```python
from build123d import *

# Parameters (mm, degrees)
SKETCH_1_R          = 5
EXTRUDE_1_DEPTH     = 14
SKETCH_2_R          = 2.5
CUT_EXTRUDE_1_DEPTH = 7
SKETCH_3_W          = 1
SKETCH_3_H          = 14
CUT_EXTRUDE_2_DEPTH = 14
SKETCH_4_R          = 2
CUT_EXTRUDE_3_DEPTH = 10
SKETCH_5_R          = 3
CUT_EXTRUDE_4_DEPTH = 2


with BuildPart() as part:
    # 草图1 → 凸台-拉伸1 (new body)
    with BuildSketch(Plane.XY):
        Polygon((21, 0), (-21, 0), (-21, 6), (-9, 6), (-9, 32.8), (9, 32.8), (9, 6), (21, 6), align=None)
        with Locations((0, 20)):
            Circle(SKETCH_1_R, mode=Mode.SUBTRACT)
    extrude(amount=EXTRUDE_1_DEPTH)

    # 草图2 → 切除-拉伸1 (cut, through all)
    with BuildSketch(Plane(origin=(0, 6, 0), x_dir=(1, 0, 0), z_dir=(0, 1, 0))):
        with Locations((-16, -7)):
            Circle(SKETCH_2_R)
        with Locations((16, -7)):
            Circle(SKETCH_2_R)
    extrude(amount=-CUT_EXTRUDE_1_DEPTH, mode=Mode.SUBTRACT)

    # 草图3 → 切除-拉伸2 (cut)
    with BuildSketch(Plane(origin=(0, 32.8, 0), x_dir=(1, 0, 0), z_dir=(0, 1, 0))):
        with Locations((0, -7)):
            Rectangle(SKETCH_3_W, SKETCH_3_H)
    extrude(amount=-CUT_EXTRUDE_2_DEPTH, mode=Mode.SUBTRACT)

    # 草图4 → 切除-拉伸3 (cut, symmetric)
    with BuildSketch(Plane(origin=(-0.5, 0, 0), x_dir=(0, 0, -1), z_dir=(1, 0, 0))):
        with Locations((-7, 28.887468593)):
            Circle(SKETCH_4_R)
    extrude(amount=CUT_EXTRUDE_3_DEPTH, both=True, mode=Mode.SUBTRACT)

    # 草图5 → 切除-拉伸4 (cut)
    with BuildSketch(Plane(origin=(9, 0, 0), x_dir=(0, 0, -1), z_dir=(1, 0, 0))):
        with Locations((-7, 28.887468593)):
            Circle(SKETCH_5_R)
    extrude(amount=-CUT_EXTRUDE_4_DEPTH, mode=Mode.SUBTRACT)


solid = part.part
```
For this review, take the finished solid that the model builds, in its own axes (mm). A direction names the side the tool comes from. Round coordinates to 2 decimals unless told otherwise and drop trailing zeros. Write each loop counter-clockwise with the first axis right and the second up, starting at its lowest first coordinate (ties: lowest second). Pieces come first, ordered by that corner, then holes. Notation, with made-up numbers: (41.25, 17) -> (99.25, 17) arc R12 ccw to (99.25, 22) -> close; hole circle Ø3 at (-36.5, 40.25). An arc over 180 degrees is marked (long way). Use one line per item in the form item = value.
Q1. Consider section B-B (y = 20). State the section outline as (x, z) points.
Resolved:
outline = (-9, 0) -> (-5, 0) -> (-5, 14) -> (-9, 14) -> close; (5, 0) -> (9, 0) -> (9, 14) -> (5, 14) -> close
Q2. Consider section A-A (x = -16). State the section outline as (y, z) points, then the cut area to 3 significant figures.
Resolved:
outline = (0, 0) -> (6, 0) -> (6, 4.5) -> (0, 4.5) -> close; (0, 9.5) -> (6, 9.5) -> (6, 14) -> (0, 14) -> close
area = 54.0 mm²
Q3. Consider section C-C (z = 7). State how many separate pieces and enclosed holes the cut face has, then the cut area to 3 significant figures.
Resolved:
separate_pieces = 5
enclosed_holes = 0
area = 516 mm²
Q4. To check wall thickness, follow probe 1 along Z at (x, y) = (-16, 2.5); probe 2 along X at (y, z) = (20, 1.75); probe 3 along X at (y, z) = (26.5, 3.75). State the ranges of each line that lie inside material, in increasing order. Write a range as from..to.
Resolved:
probe_1 = 0..4.5, 9.5..14
probe_2 = -9..-5, 5..9
probe_3 = -9..-0.5, 0.5..9
Q5. Clearance check with flat-ended pins moving along their axes: pin 1 Ø6.5 at (y, z) = (28.89, 7) entering from -X; pin 2 Ø6 at (y, z) = (10.5, 5.5) entering from +X; pin 3 Ø3 at (y, z) = (29.5, 6) entering from +X; pin 4 Ø3.5 at (y, z) = (28.89, 7) entering from -X. State where each tip first meets the part, or that it passes through.
Resolved:
pin_1 = -9
pin_2 = 9
pin_3 = 7
pin_4 = through
Q6. Consider section D-D (x = -2). State the section outline as (y, z) points, then the cut area to 3 significant figures.
Resolved:
outline = (0, 0) -> (15.42, 0) -> (15.42, 14) -> (0, 14) -> close; (24.58, 0) -> (32.8, 0) -> (32.8, 14) -> (24.58, 14) -> close; hole circle Ø4 at (28.89, 7)
area = 318 mm²
Q7. Machinability: for faces 1 (the flat face through (-9, 19, 7)), 2 (the flat face through (-0.5, 27, 9)), 3 (the flat face through (13.6, 6, 8.5)), which of the approach directions +Z, -Z, +X, -X, +Y, -Y give a long, thin tool a straight path to every point of the face, cutting with its end or side? Answer none if there is none.
Resolved:
face_1 = +Z, -Z, -X, +Y
face_2 = +Z, -Z, +Y
face_3 = +Z, -Z, +X, +Y
Q8. The part is to be moulded in two halves that separate along Y. For faces 4 (the flat face through (0, 9, 14)), 5 (the cylindrical face through (0, 15, 7)), 6 (the flat face through (-5, 32.8, 7)), say which applies: released by +Y, released by -Y, zero draft, split by the parting line, or undercut.
Resolved:
face_4 = zero draft
face_5 = undercut
face_6 = released by +Y
